Input: part model. Units: mm. Frame: model coordinates. Coordinates: 2 decimals unless noted, no trailing zeros. Loops run counter-clockwise (first coordinate to the right, second up) from the corner with the lowest first, then second, coordinate; pieces in that order, holes last.
```python
from build123d import *

# Parameters (mm, degrees)
SKETCH1_R           = 85
SKETCH1_R_2         = 60
BOSS_EXTRUDE1_DEPTH = 12.2
FILLET1_R           = 1.1


with BuildPart() as part:
    # Sketch1 → Boss-Extrude1 (new body)
    with BuildSketch(Plane(origin=(0, 0, 0), x_dir=(1, 0, 0), z_dir=(0, 1, 0))):
        Circle(SKETCH1_R)
        Circle(SKETCH1_R_2, mode=Mode.SUBTRACT)
    extrude(amount=BOSS_EXTRUDE1_DEPTH)

    # Fillet1
    fillet1_edges = [part.edges().sort_by_distance(p)[0] for p in [
        (-85, 12.2, 0),
        (-60, 12.2, 0),
    ]]
    fillet(fillet1_edges, radius=FILLET1_R)

    # Sketch2 → Cut-Revolve1 (revolve, cut)
    with BuildSketch(Plane.XY):
        with BuildLine():
            Line((-77.98, 0), (-67.02, 0))
            ThreePointArc((-67.02, 0), (-72.5, 1.827500428), (-77.98, 0))
        make_face()
    revolve(axis=Axis((0, 11.1, 0), (0, -1, 0)), mode=Mode.SUBTRACT)


solid = part.part
```
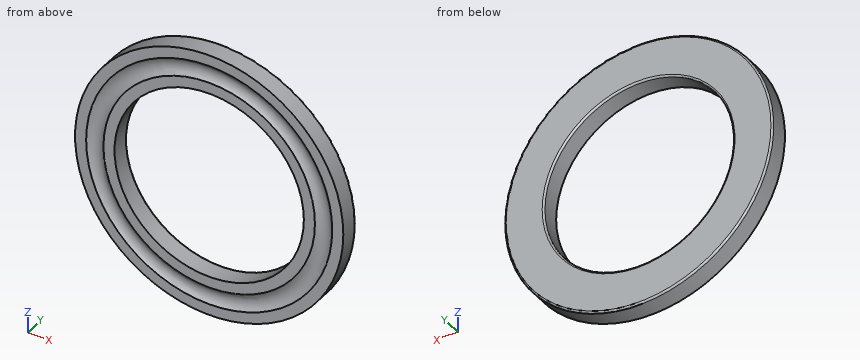
Item 1: Section query A-A (z = 0). Output: boundary loops of the cut face in (x, y), then the cut area to 3 significant figures.
Result:
outline: (-85, 0) - (-77.98, 0) arc R9.13 cw to (-67.02, 0) - (-60, 0) - (-60, 11.1) arc R1.1 ccw to (-61.1, 12.2) - (-83.9, 12.2) arc R1.1 ccw to (-85, 11.1) - close; (60, 0) - (67.02, 0) arc R9.13 cw to (77.98, 0) - (85, 0) - (85, 11.1) arc R1.1 ccw to (83.9, 12.2) - (61.1, 12.2) arc R1.1 ccw to (60, 11.1) - close
area: 582 mm2
Item 2: Line query: L1, parallel to Z at x = 0, y = 8.5; L2, parallel to X at y = 1, z = 1.5. Output: solid intervals per line, ascending.
Result:
L1: z = -85 to -60, 60 to 85
L2: x = -84.99 to -76.28, -68.69 to -59.98, 59.98 to 68.69, 76.28 to 84.99
Item 3: Section query B-B (x = 0). Output: boundary loops of the cut face in (y, z).
Result:
outline: (0, -85) - (11.1, -85) arc R1.1 ccw to (12.2, -83.9) - (12.2, -61.1) arc R1.1 ccw to (11.1, -60) - (0, -60) - (0, -67.02) arc R9.13 cw to (0, -77.98) - close; (0, 60) - (11.1, 60) arc R1.1 ccw to (12.2, 61.1) - (12.2, 83.9) arc R1.1 ccw to (11.1, 85) - (0, 85) - (0, 77.98) arc R9.13 cw to (0, 67.02) - close
Item 4: Section query C-C (y = 4). Output: boundary loops of the cut face in (x, z), then the cut area to 3 significant figures.
Result:
outline: circle Ø170 at (0, 0); hole circle Ø120 at (0, 0)
area: 11,400 mm2
Item 5: Contact query for flat-ended pins moving along their axis: P1, Ø1, axis at x = 22, y = 1.5, coming from the -Z side; P2, Ø4, axis at x = -33.5, y = 7.5, coming from the -Z side; P3, Ø6, axis at y = 6.5, z = 9.5, coming from the +X side. Output: stop coordinate, or through.
Result:
P1: stops at z = -82.24
P2: stops at z = -78.95
P3: stops at x = 84.75
